Here's how the part is built. I have some questions about the finished solid (model axes, mm). Face numbers are marked on the shaded views. A direction names the side the tool comes from. Round coordinates to 2 decimals unless told otherwise and drop trailing zeros. Write each loop counter-clockwise with the first axis right and the second up, starting at its lowest first coordinate (ties: lowest second). Pieces come first, ordered by that corner, then holes. Notation, with made-up numbers: (-1.75, 63.5) - (21.25, 63.5) arc R23 ccw to (21.25, 93.5) - close; hole circle Ø1 at (29, 38). An arc over 180 degrees is marked (long way). One line per question, with ' | ' between items. Start each with the question number.
(1) Imagine slicing it at A-A (z = 30). Write out the boundary of the cut face in (x, y), plus the area to 3 significant figures.
(2) If I drill on L1, parallel to X at y = 1.4, z = 10; L2, parallel to X at y = 21, z = -9.5; L3, parallel to Z at x = -6, y = 1, over which ranges is the centre line in solid material (lowest first)?
(3) Imagine slicing it at D-D (z = 19.5). Write out the boundary of the cut face in (x, y), plus the area to 3 significant figures.
(4) Imagine slicing it at C-C (x = 0.75). Write out the boundary of the cut face in (y, z).
(5) Imagine slicing it at B-B (y = 12). Write out the boundary of the cut face in (x, z).
(6) Thinking about a two-plate mould opening in Z: for the marked faces 1, 2, 3 and 4, which applies, pulls with the +Z half, pulls with the -Z half, needs draft (parallel to the pull), parting line crosses it, or undercut?
(7) For the marked faces 5, 6, 7 and 8, which set-ups out of +Z, -Z, +X, -X, +Y, -Y let a thin tool reach every point of the face, with its end or its side?
(8) Will these pins go through, and if not, where does the flat tip stop? pin 1 (3.5 mm diameter, centred on x = -5, y = 6, fed in from -Z); pin 2 (4 mm diameter, centred on x = 5, y = 6, fed in from +Z); pin 3 (2.5 mm diameter, centred on x = -5, y = 21, fed in from +Z); pin 4 (6 mm diameter, centred on x = -7.5, z = 27, fed in from +Y).
from build123d import *

# Parameters (mm, degrees)
EXTRUDE_1_DEPTH          = 10
RIB_1_REACH              = 49.707
SKETCH_3_WALL_W          = 139.958978308
SKETCH_3_WALL_H          = 3
EXTRUDE_2_DEPTH          = 20
CUT_EXTRUDE_1_DEPTH      = 46.221676218
CUT_EXTRUDE_1_DEPTH_BACK = 46.221676218
SKETCH_4_R               = 1.6
FILLET_1_R               = 1
CUT_EXTRUDE_2_DEPTH      = 47.270941205
CUT_EXTRUDE_2_DEPTH_BACK = 47.270941205
SKETCH_6_R               = 1.6
FILLET_2_R               = 0.5
FILLET_START             = 2.5
FILLET_3_3_DEPTH         = 8.5
FILLET_START_2           = -11
FILLET_3_4_DEPTH         = 8.5
FILLET_START_3           = -2.5
FILLET_3_5_DEPTH         = 5
CUT_EXTRUDE_3_DEPTH      = 1


with BuildPart() as part:
    # 草图1 → 凸台-拉伸1 (new, symmetric)
    with BuildSketch(Plane(origin=(0, 0, 0), x_dir=(0, 0, -1), z_dir=(1, 0, 0))):
        Polygon((0, 24), (0, 0), (-40, 0), (-40, 3), (-3, 3), (-3, 24), align=None)
    extrude(amount=EXTRUDE_1_DEPTH, both=True)

    # 草图3 wall → 筋1 (add, up to next)
    with BuildSketch(Plane(origin=(0, 13.5, 21.5), x_dir=(0, -0.493605519458, 0.869685915236), z_dir=(0, -0.869685915236, -0.493605519458)), mode=Mode.PRIVATE) as rib_1_sk1:
        Rectangle(SKETCH_3_WALL_W, SKETCH_3_WALL_H)
    rib_1_tool1 = extrude(rib_1_sk1.sketch, amount=RIB_1_REACH, mode=Mode.PRIVATE) - part.part
    add(rib_1_tool1.solids().sort_by_distance((0, 13.5, 21.5))[0])

    # 草图5 → 凸台-拉伸2 (add)
    with BuildSketch(Plane.ZY.offset(10)):
        Polygon((0, 0), (-11.5, 0), (-11.5, 3), (-11.5, 24), (-8.5, 24), (-8.5, 3), (0, 3), align=None)
    extrude(amount=-EXTRUDE_2_DEPTH)

    # 草图4 → 切除-拉伸1 (cut, two sides: drawn at the far end of the back side and taken through both)
    with BuildSketch(Plane.XY.offset(3).offset(-CUT_EXTRUDE_1_DEPTH_BACK)):
        with Locations((-5, 21)):
            Circle(SKETCH_4_R)
        with Locations((-5, 6)):
            Circle(SKETCH_4_R)
        with Locations((5, 21)):
            Circle(SKETCH_4_R)
        with Locations((5, 6)):
            Circle(SKETCH_4_R)
    extrude(amount=CUT_EXTRUDE_1_DEPTH + CUT_EXTRUDE_1_DEPTH_BACK, mode=Mode.SUBTRACT)

    # 圆角1
    fillet_1_edges = [part.edges().sort_by_distance(p)[0] for p in [
        (5.75, 3, 3),
        (-5.75, 3, 3),
        (-1.5, 13.5, 3),
        (-1.5, 3, 21.5),
        (1.5, 13.5, 3),
        (1.5, 3, 21.5),
    ]]
    fillet(fillet_1_edges, radius=FILLET_1_R)

    # 草图6 → 切除-拉伸2 (cut, two sides: drawn at the far end of the back side and taken through both)
    with BuildSketch(Plane(origin=(0, 3, 0), x_dir=(1, 0, 0), z_dir=(0, 1, 0)).offset(-CUT_EXTRUDE_2_DEPTH_BACK)):
        with Locations(Location((-6, -10, 0), (0, 0, 270))):
            Circle(SKETCH_6_R)
        with Locations(Location((6, -10, 0), (0, 0, 270))):
            Circle(SKETCH_6_R)
        with Locations(Location((-6, -30, 0), (0, 0, 270))):
            Circle(SKETCH_6_R)
        with Locations(Location((6, -30, 0), (0, 0, 270))):
            Circle(SKETCH_6_R)
    extrude(amount=CUT_EXTRUDE_2_DEPTH + CUT_EXTRUDE_2_DEPTH_BACK, mode=Mode.SUBTRACT)

    # 圆角2
    fillet_2_edges = [part.edges().sort_by_distance(p)[0] for p in [
        (6, 3, 8.4),
        (-6, 3, 28.4),
        (6, 3, 28.4),
        (-6, 3, 8.4),
    ]]
    fillet(fillet_2_edges, radius=FILLET_2_R)

    # 圆角3: read off the stored shape, not the designer's step
    # 圆角3 outline → 圆角3 (revolve, cut)
    with BuildSketch(Plane(origin=(-2.5, 0, 4), x_dir=(1, 0, 0), z_dir=(0, 0, 1))):
        with BuildLine():
            Line((1, 24), (1, 23.5))
            ThreePointArc((1, 23.5), (1.146446609, 23.853553391), (1.5, 24))
            Line((1.5, 24), (1, 24))
        make_face()
    revolve(axis=Axis((-2.5, 0, 4), (0, 1, 0)), mode=Mode.SUBTRACT)

    # Fillet 3 2 outline → Fillet 3 2 (revolve, cut)
    with BuildSketch(Plane(origin=(2.5, 0, 4), x_dir=(1, 0, 0), z_dir=(0, 0, 1))):
        with BuildLine():
            Line((1, 24), (1, 23.5))
            ThreePointArc((1, 23.5), (1.146446609, 23.853553391), (1.5, 24))
            Line((1.5, 24), (1, 24))
        make_face()
    revolve(axis=Axis((2.5, 0, 4), (0, 1, 0)), mode=Mode.SUBTRACT)

    # Fillet 3 3 outline → Fillet 3 3 (cut)
    with BuildSketch(Plane.YZ.offset(FILLET_START)):
        with BuildLine():
            ThreePointArc((23.5, 3), (23.853553391, 2.853553391), (24, 2.5))
            Line((24, 2.5), (24, 3))
            Line((24, 3), (23.5, 3))
        make_face()
    extrude(amount=FILLET_3_3_DEPTH, mode=Mode.SUBTRACT)

    # Fillet 3 4 outline → Fillet 3 4 (cut)
    with BuildSketch(Plane.YZ.offset(FILLET_START_2)):
        with BuildLine():
            ThreePointArc((23.5, 3), (23.853553391, 2.853553391), (24, 2.5))
            Line((24, 2.5), (24, 3))
            Line((24, 3), (23.5, 3))
        make_face()
    extrude(amount=FILLET_3_4_DEPTH, mode=Mode.SUBTRACT)

    # Fillet 3 5 outline → Fillet 3 5 (cut)
    with BuildSketch(Plane.YZ.offset(FILLET_START_3)):
        with BuildLine():
            Line((24, 2.867997744), (24, 3))
            Line((24, 3), (23.934842958, 3.114800503))
            ThreePointArc((23.934842958, 3.114800503), (23.983436386, 2.995627131), (24, 2.867997744))
        make_face()
    extrude(amount=FILLET_3_5_DEPTH, mode=Mode.SUBTRACT)

    # 草图7 → 切除-拉伸3 (cut)
    with BuildSketch(Plane(origin=(0, 0, -11.5), x_dir=(-1, 0, 0), z_dir=(0, 0, -1))):
        Polygon((-5, 8.8), (-7.424871131, 7.4), (-7.424871131, 4.6), (-5, 3.2), (-2.575128869, 4.6), (-2.575128869, 7.4), align=None)
        Polygon((-5, 23.8), (-7.424871131, 22.4), (-7.424871131, 19.6), (-5, 18.2), (-2.575128869, 19.6), (-2.575128869, 22.4), align=None)
        Polygon((5, 23.8), (2.575128869, 22.4), (2.575128869, 19.6), (5, 18.2), (7.424871131, 19.6), (7.424871131, 22.4), align=None)
        Polygon((5, 8.8), (2.575128869, 7.4), (2.575128869, 4.6), (5, 3.2), (7.424871131, 4.6), (7.424871131, 7.4), align=None)
    extrude(amount=-CUT_EXTRUDE_3_DEPTH, mode=Mode.SUBTRACT)


solid = part.part
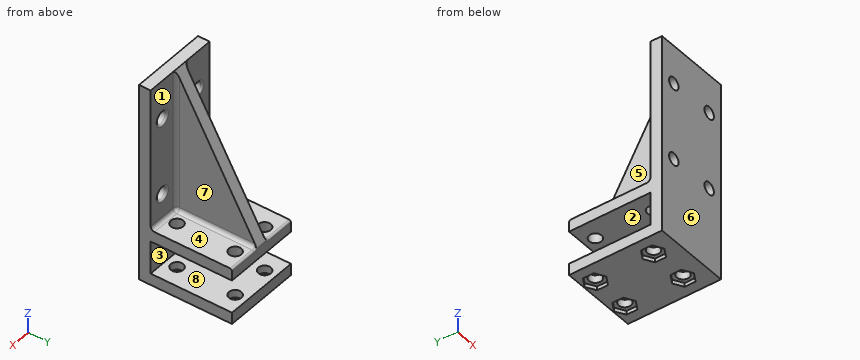
Check sheet entries:
1) outline: (-10, 0) - (-7.6, 0) - (-7.6, 2.5) arc R0.5 ccw to (-8.1, 3) - (-10, 3) - close; (-4.4, 0) - (4.4, 0) - (4.4, 2.5) arc R0.5 ccw to (3.9, 3) - (2.5, 3) arc R1 cw to (1.5, 4) - (1.5, 8.68) - (-1.5, 8.68) - (-1.5, 4) arc R1 cw to (-2.5, 3) - (-3.9, 3) arc R0.5 ccw to (-4.4, 2.5) - close; (7.6, 0) - (10, 0) - (10, 3) - (8.1, 3) arc R0.5 ccw to (7.6, 2.5) - close | area: 58.0 mm^2
2) L1: -10 to -7.6, -4.4 to 4.4, 7.6 to 10 | L2: -10 to -6.6, -3.4 to 3.4, 6.6 to 10 | L3: -11.5 to 8.4, 11.6 to 28.4, 31.6 to 40
3) outline: (-10, 0) - (10, 0) - (10, 3) - (2.5, 3) arc R1 cw to (1.5, 4) - (1.5, 14.64) - (-1.5, 14.64) - (-1.5, 4) arc R1 cw to (-2.5, 3) - (-10, 3) - close | area: 95.3 mm^2
4) outline: (0, -11.5) - (24, -11.5) - (24, -8.5) - (3, -8.5) - (3, 0) - (24, 0) - (24, 2.87) arc R0.5 ccw to (23.93, 3.11) - (3, 40) - (0, 40) - close
5) outline: (-10, -11.5) - (10, -11.5) - (10, -8.5) - (-10, -8.5) - close; (-10, 0) - (10, 0) - (10, 3) - (2.5, 3) arc R1 cw to (1.5, 4) - (1.5, 24.14) - (-1.5, 24.14) - (-1.5, 4) arc R1 cw to (-2.5, 3) - (-10, 3) - close
6) face 1: needs draft | face 2: undercut | face 3: undercut | face 4: pulls with the +Z half
7) face 5: +Z, -X, +Y | face 6: +Z, -Z, +X, -X, -Y | face 7: +Z, +X, +Y | face 8: +X, -X, +Y
8) pin 1: z = -10.5 | pin 2: z = 3 | pin 3: through | pin 4: y = 3
